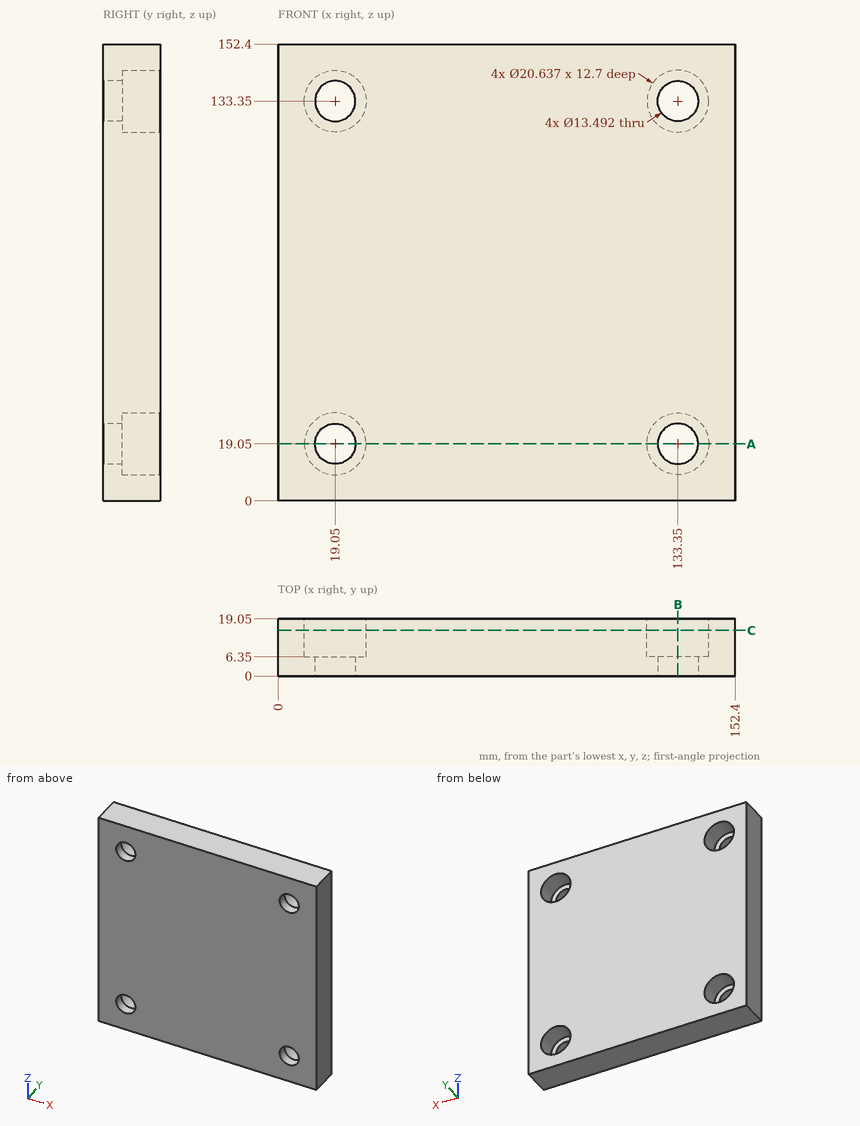
The figure shows three views and two pictorial views of one solid part (mm, origin at its lowest corner). Answer the questions. Coordinates: 2 decimals unless noted, no trailing zeros. Order: outer loops, then holes, each group sorted by start corner. A loop starts at its lowest first (then second) coordinate and runs counter-clockwise, first axis right, second up. Notation, with made-up numbers: (-32.75, 18) - (-23.75, 18) arc R9 cw to (-23.75, 30) - close; hole circle Ø5 at (85.5, 2). An arc over 180 degrees is marked (long way). Answer as a JSON object with one key per item and string values.
1. Find section A-A on z = 19.05. Determine the outline of the cut face in (x, y).
Output values:
{"outline": "(0, 0) - (12.3, 0) - (12.3, 6.35) - (8.73, 6.35) - (8.73, 19.05) - (0, 19.05) - close; (25.8, 0) - (126.6, 0) - (126.6, 6.35) - (123.03, 6.35) - (123.03, 19.05) - (29.37, 19.05) - (29.37, 6.35) - (25.8, 6.35) - close; (140.1, 0) - (152.4, 0) - (152.4, 19.05) - (143.67, 19.05) - (143.67, 6.35) - (140.1, 6.35) - close"}
2. Each of these flat-tipped pins is pushed along its axis until it touches: P1, Ø21.5, axis at x = 19.05, z = 19.05, coming from the -Y side; P2, Ø6, axis at x = 130.5, z = 129.5, coming from the +Y side. Where does it stop, or does it pass through?
Output values:
{"P1": "stops at y = 0", "P2": "stops at y = 6.35"}
3. Find section C-C on y = 15.25. Determine the outline of the cut face in (x, z), plus the area to 3 significant figures.
Output values:
{"outline": "(0, 0) - (152.4, 0) - (152.4, 152.4) - (0, 152.4) - close; hole circle Ø20.64 at (19.05, 19.05); hole circle Ø20.64 at (19.05, 133.35); hole circle Ø20.64 at (133.35, 19.05); hole circle Ø20.64 at (133.35, 133.35)", "area": "21,900 mm²"}
4. Consider line 1 (Z direction, x = 19.05, y = 9.25); line 2 (Z direction, x = 19.05, y = 2); line 3 (Y direction, x = 28, z = 130). Determine where each line is inside the solid, lowest interval first.
Output values:
{"line 1": "z = 0 to 8.73, 29.37 to 123.03, 143.67 to 152.4", "line 2": "z = 0 to 12.3, 25.8 to 126.6, 140.1 to 152.4", "line 3": "y = 0 to 6.35"}
5. Find section B-B on x = 133.35. Determine the outline of the cut face in (y, z), plus the area to 3 significant figures.
Output values:
{"outline": "(0, 0) - (19.05, 0) - (19.05, 8.73) - (6.35, 8.73) - (6.35, 12.3) - (0, 12.3) - close; (0, 25.8) - (6.35, 25.8) - (6.35, 29.37) - (19.05, 29.37) - (19.05, 123.03) - (6.35, 123.03) - (6.35, 126.6) - (0, 126.6) - close; (0, 140.1) - (6.35, 140.1) - (6.35, 143.67) - (19.05, 143.67) - (19.05, 152.4) - (0, 152.4) - close", "area": "2,210 mm²"}
